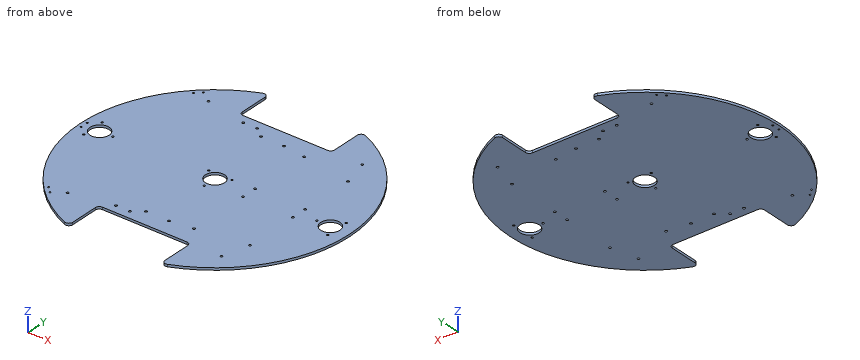
from build123d import *

# Parameters (mm, degrees)
SKETCH_1_R           = 175
EXTRUDE_1_DEPTH      = 3
CUT_EXTRUDE_1_DEPTH  = 3
FILLET_1_R           = 5
FILLET_2_R           = 5
FILLET_3_R           = 5
SKETCH_5_R           = 1.5
CUT_EXTRUDE_4_DEPTH  = 3
SKETCH_10_R          = 12.5
SKETCH_10_R_2        = 1.3
CUT_EXTRUDE_13_DEPTH = 10
SKETCH_14_R          = 1.1
CUT_EXTRUDE_14_DEPTH = 10
SKETCH_12_R          = 1.5
CUT_EXTRUDE_17_DEPTH = 10
SKETCH_13_R          = 1.5
CUT_EXTRUDE_18_DEPTH = 5
SKETCH_15_R          = 1.5
CUT_EXTRUDE_19_DEPTH = 4


with BuildPart() as part:
    # ｽｹｯﾁ1 → ﾎﾞｽ - 押し出し1 (new body)
    with BuildSketch(Plane.XY):
        Circle(SKETCH_1_R)
    extrude(amount=EXTRUDE_1_DEPTH)

    # ｽｹｯﾁ2 → ｶｯﾄ - 押し出し1 (cut)
    with BuildSketch(Plane.XY.offset(3)):
        with BuildLine():
            Line((-60, 115), (0, 115))
            Line((0, 115), (0, 175))
            ThreePointArc((0, 175), (-30.465194158, 172.327803749), (-60, 164.392822228))
            Line((-60, 164.392822228), (-60, 115))
        make_face()
        with BuildLine():
            Line((0, 175), (0, 115))
            Line((0, 115), (60, 115))
            Line((60, 115), (60, 164.392822228))
            ThreePointArc((60, 164.392822228), (30.465194158, 172.327803749), (0, 175))
        make_face()
        with BuildLine():
            Line((0, -175), (0, -115))
            Line((0, -115), (-60, -115))
            Line((-60, -115), (-60, -164.392822228))
            ThreePointArc((-60, -164.392822228), (-30.465194158, -172.327803749), (0, -175))
        make_face()
        with BuildLine():
            Line((60, -115), (0, -115))
            Line((0, -115), (0, -175))
            ThreePointArc((0, -175), (30.465194158, -172.327803749), (60, -164.392822228))
            Line((60, -164.392822228), (60, -115))
        make_face()
    extrude(amount=-CUT_EXTRUDE_1_DEPTH, mode=Mode.SUBTRACT)

    # ﾌｨﾚｯﾄ1
    fillet_1_edges = [part.edges().sort_by_distance(p)[0] for p in [
        (-60, 164.392822228, 1.5),
    ]]
    fillet(fillet_1_edges, radius=FILLET_1_R)

    # ﾌｨﾚｯﾄ2
    fillet_2_edges = [part.edges().sort_by_distance(p)[0] for p in [
        (-60, 115, 1.5),
        (60, 164.392822228, 1.5),
        (60, 115, 1.5),
    ]]
    fillet(fillet_2_edges, radius=FILLET_2_R)

    # ﾌｨﾚｯﾄ3
    fillet_3_edges = [part.edges().sort_by_distance(p)[0] for p in [
        (-60, -115, 1.5),
        (60, -115, 1.5),
        (60, -164.392822228, 1.5),
        (-60, -164.392822228, 1.5),
    ]]
    fillet(fillet_3_edges, radius=FILLET_3_R)

    # ｽｹｯﾁ5 → ｶｯﾄ - 押し出し4 (cut)
    with BuildSketch(Plane.XY.offset(3)):
        with Locations((-100, -115)):
            Circle(SKETCH_5_R)
        with Locations((100, -115)):
            Circle(SKETCH_5_R)
        with Locations((100, 115)):
            Circle(SKETCH_5_R)
        with Locations((-100, 115)):
            Circle(SKETCH_5_R)
    extrude(amount=-CUT_EXTRUDE_4_DEPTH, mode=Mode.SUBTRACT)

    # ｽｹｯﾁ10 → ｶｯﾄ - 押し出し13 (cut)
    with BuildSketch(Plane.XY.offset(3)):
        with Locations((-150, 0)):
            Circle(SKETCH_10_R)
        with Locations((150, 0)):
            Circle(SKETCH_10_R)
        Circle(SKETCH_10_R)
        with Locations((132.5, 0)):
            Circle(SKETCH_10_R_2)
        with Locations((158.75, 15.155444566)):
            Circle(SKETCH_10_R_2)
        with Locations((158.75, -15.155444566)):
            Circle(SKETCH_10_R_2)
        with Locations((-15.155444566, 8.75)):
            Circle(SKETCH_10_R_2)
        with Locations((15.155444566, 8.75)):
            Circle(SKETCH_10_R_2)
        with Locations((0, -17.5)):
            Circle(SKETCH_10_R_2)
        with Locations((-158.75, 15.155444566)):
            Circle(SKETCH_10_R_2)
        with Locations((-158.75, -15.155444566)):
            Circle(SKETCH_10_R_2)
        with Locations((-132.632898389, 0)):
            Circle(SKETCH_10_R_2)
    extrude(amount=-CUT_EXTRUDE_13_DEPTH, mode=Mode.SUBTRACT)

    # ｽｹｯﾁ14 → ｶｯﾄ - 押し出し14 (cut)
    with BuildSketch(Plane.XY.offset(3)):
        with Locations((-170, 5)):
            Circle(SKETCH_14_R)
        with Locations((-170, -5)):
            Circle(SKETCH_14_R)
        with Locations((-114.933514447, 125.360628815)):
            Circle(SKETCH_14_R)
        with Locations((-122.102620524, 118.388977786)):
            Circle(SKETCH_14_R)
        with Locations((-122.102620524, -118.388977786)):
            Circle(SKETCH_14_R)
        with Locations((-114.933514447, -125.360628815)):
            Circle(SKETCH_14_R)
    extrude(amount=-CUT_EXTRUDE_14_DEPTH, mode=Mode.SUBTRACT)

    # ｽｹｯﾁ12 → ｶｯﾄ - 押し出し17 (cut)
    with BuildSketch(Plane.XY.offset(3)):
        with Locations((-15, 94)):
            Circle(SKETCH_12_R)
        with Locations((15, 94)):
            Circle(SKETCH_12_R)
        with Locations((-15, -94)):
            Circle(SKETCH_12_R)
        with Locations((15, -94)):
            Circle(SKETCH_12_R)
    extrude(amount=-CUT_EXTRUDE_17_DEPTH, mode=Mode.SUBTRACT)

    # ｽｹｯﾁ13 → ｶｯﾄ - 押し出し18 (cut)
    with BuildSketch(Plane.XY.offset(3)):
        with Locations((-28, -104)):
            Circle(SKETCH_13_R)
        with Locations((-46, -104)):
            Circle(SKETCH_13_R)
        with Locations((-46, 104)):
            Circle(SKETCH_13_R)
        with Locations((-28, 104)):
            Circle(SKETCH_13_R)
    extrude(amount=-CUT_EXTRUDE_18_DEPTH, mode=Mode.SUBTRACT)

    # ｽｹｯﾁ15 → ｶｯﾄ - 押し出し19 (cut, through all)
    with BuildSketch(Plane.XY.offset(3)):
        with Locations((44.252990552, 10)):
            Circle(SKETCH_15_R)
        with Locations((44.252990552, 90)):
            Circle(SKETCH_15_R)
        with Locations((109.252990552, 10)):
            Circle(SKETCH_15_R)
        with Locations((109.252990552, 80)):
            Circle(SKETCH_15_R)
        with Locations((44.252990552, -10)):
            Circle(SKETCH_15_R)
        with Locations((109.252990552, -10)):
            Circle(SKETCH_15_R)
        with Locations((44.252990552, -90)):
            Circle(SKETCH_15_R)
        with Locations((109.252990552, -80)):
            Circle(SKETCH_15_R)
    extrude(amount=-CUT_EXTRUDE_19_DEPTH, mode=Mode.SUBTRACT)


solid = part.part
Could you check a few things on this model? Use its own coordinates, in mm. Round coordinates to 2 decimals unless told otherwise and drop trailing zeros. Order: outer loops, then holes, each group sorted by start corner. A loop starts at its lowest first (then second) coordinate and runs counter-clockwise, first axis right, second up.
(1) Imagine slicing it at A-A (x = -150). Write out the boundary of the cut face in (y, z).
Response values:
outline: (-90.14, 0) - (-12.5, 0) - (-12.5, 3) - (-90.14, 3) - close; (12.5, 0) - (90.14, 0) - (90.14, 3) - (12.5, 3) - close
(2) Imagine slicing it at C-C (y = -31). Write out the boundary of the cut face in (x, z).
Response values:
outline: (-172.23, 0) - (172.23, 0) - (172.23, 3) - (-172.23, 3) - close
(3) Please list where these lines run through material, in increasing order: line 1 along Y through (x, z) = (-15, 1.8); line 2 along Y through (x, z) = (-28, 1.7); line 3 along Y through (x, z) = (14, 0.9).
Response values:
line 1: y = -115 to -95.5, -92.5 to 7.46, 10.04 to 92.5, 95.5 to 115
line 2: y = -115 to -105.5, -102.5 to 102.5, 105.5 to 115
line 3: y = -115 to -95.12, -92.88 to 8.15, 9.35 to 92.88, 95.12 to 115
(4) Imagine slicing it at B-B (x = -22.5). Write out the boundary of the cut face in (y, z).
Response values:
outline: (-115, 0) - (115, 0) - (115, 3) - (-115, 3) - close
(5) Imagine slicing it at D-D (z = 0.85). Count the separate pieces of the cut face and the enclosed holes in it, plus the area to 3 significant figures.
Response values:
separate pieces: 1
enclosed holes: 38
area: 80,900 mm2
(6) I'm going to push flat-ended pins straight in: pin 1 (1.6 mm diameter, centred on x = 158.75, y = 15.16, fed in from +Z); pin 2 (0.9 mm diameter, centred on y = 140.5, z = 2, fed in from -X). Where does each tip first touch, or does it pass through?
Response values:
pin 1: passes through
pin 2: stops at x = -104.93
